Read the model definition and answer for the solid it produces. Units are mm, in the model's axes. A direction names the side the tool comes from. Give positions to 0.01 mm unless a question says otherwise; leave off trailing zeros. Loops run counter-clockwise (first coordinate to the right, second up) from the corner with the lowest first, then second, coordinate; pieces in that order, holes last. Notation, with made-up numbers: (-22, 34) - (7, 34) arc R24 cw to (7, 64) - close; hole circle Ø4 at (32.25, 28). An arc over 180 degrees is marked (long way). Put each result on its own line as item: value. Start each with the question number.
1. A cutting plane is placed at A-A, the plane z = 23. Count the separate pieces of the cut face and the enclosed holes in it, plus the area to 3 significant figures.
2. Given pin 1 Ø4.5 at (x, y) = (15, 5.1) entering from +Z; pin 2 Ø2 at (x, y) = (0, 20.1) entering from +Z; pin 3 Ø5 at (x, z) = (19, 12.5) entering from +Y; pin 4 Ø6 at (x, z) = (-22, 11) entering from -Y, each flat-ended and moving along its own axis, determine where each tip first touches the part or whether it passes through.
3. A cutting plane is placed at B-B, the plane x = -15. Determine the outline of the cut face in (y, z), plus the area to 3 significant figures.
4. For faces 4 (the flat face through (-9.1, -15, 12)), 5 (the cylindrical face through (26.4, 5.23, 0.94)), 6 (the flat face through (-9.1, 25, 12)), 7 (the flat face through (18, 10.2, 13)), determine the directions among +Z, -Z, +X, -X, +Y, -Y from which every point of the face is accessible in a straight line to the end or side of a thin tool.
5. A cutting plane is placed at D-D, the plane y = 20.1. Determine the outline of the cut face in (x, z).
6. For a pull along X with two mould halves and no side action, classify faces 1 (the flat face through (28.484, 12, 12)), 2 (the flat face through (0, 3, 2)), 3 (the flat face through (-20, -4, 12)) as released by +X, released by -X, zero draft, split by the parting line, or undercut.
7. A cutting plane is placed at C-C, the plane y = 5.1. Determine the outline of the cut face in (x, z), plus the area to 3 significant figures.
8. Consider L1, parallel to Y at x = -14.5, z = 9; L2, parallel to X at y = 24, z = 13; L3, parallel to X at y = 20.1, z = 1.65. Determine where each line is inside the solid, lowest interval first. Write a range as from..to.
```python
from build123d import *

# Parameters (mm, degrees)
F1_DEPTH       = 2
F2_DEPTH       = 25
F3_R           = 2
F4_T1_DEPTH    = 4
F4_T3_DEPTH    = 4
F4_T5_DEPTH    = 4
F4_T7_DEPTH    = 18.2
F4_T9_DEPTH    = 18.2
F4_T11_DEPTH   = 4
F5_R           = 2
F6_SIZE        = 2
F8_D           = 3.3
F8_CSINK_D     = 6
F8_CSINK_ANGLE = 90


# Not quite as in the source:
# - a fillet or chamfer that OpenCascade refuses, or shapes differently, is made with other operations: its cross-section is extruded or revolved along the edge and cut away or added
# - a feature names something its author has since deleted; it is built from what else it names


with BuildPart() as f1:
    # F0 (on Top) → F1 (new body)
    with BuildSketch(Plane.XY):
        Polygon((28.4836267311, 0), (28.4836267311, 10.2), (5.1, 10.2), (5.1, 33.5836267311), (-5.1, 33.5836267311), (-5.1, 10.2), (-28.4836267311, 10.2), (-28.4836267311, 0), (-5.1, 0), (-5.1, -23.3836267311), (5.1, -23.3836267311), (5.1, 0), align=None)
        Polygon((5.1, 10.2), (28.4836267311, 10.2), (28.4836267311, 14.2), (9.1, 14.2), (9.1, 33.5836267311), (5.1, 33.5836267311), align=None)
        Polygon((28.4836267311, -4), (28.4836267311, 0), (5.1, 0), (5.1, -23.3836267311), (9.1, -23.3836267311), (9.1, -4), align=None)
        Polygon((-5.1, 10.2), (-5.1, 33.5836267311), (-9.1, 33.5836267311), (-9.1, 14.2), (-28.4836267311, 14.2), (-28.4836267311, 10.2), align=None)
        Polygon((-9.1, -23.3836267311), (-5.1, -23.3836267311), (-5.1, 0), (-28.4836267311, 0), (-28.4836267311, -4), (-9.1, -4), align=None)
    extrude(amount=F1_DEPTH)

    # F0 (on Top) → F2 (join)
    with BuildSketch(Plane.XY):
        Polygon((-5.1, 10.2), (-5.1, 33.5836267311), (-9.1, 33.5836267311), (-9.1, 14.2), (-28.4836267311, 14.2), (-28.4836267311, 10.2), align=None)
        Polygon((5.1, 10.2), (28.4836267311, 10.2), (28.4836267311, 14.2), (9.1, 14.2), (9.1, 33.5836267311), (5.1, 33.5836267311), align=None)
        Polygon((-9.1, -23.3836267311), (-5.1, -23.3836267311), (-5.1, 0), (-28.4836267311, 0), (-28.4836267311, -4), (-9.1, -4), align=None)
        Polygon((28.4836267311, -4), (28.4836267311, 0), (5.1, 0), (5.1, -23.3836267311), (9.1, -23.3836267311), (9.1, -4), align=None)
    extrude(amount=F2_DEPTH)

    # F3
    f3_edges = [f1.edges().sort_by_distance(p)[0] for p in [
        (9.1, 14.2, 12.5),
        (9.1, -4, 12.5),
    ]]
    fillet(f3_edges, radius=F3_R)

    # F4: fillet of radius 5 on 12 edges, made by hand

    # F4_s2 → F4_t1 (cut)
    with BuildSketch(Plane.XZ.offset(-14.2)):
        with BuildLine():
            ThreePointArc((23.4836267311, 25), (27.0191606371, 23.5355339059), (28.4836267311, 20))
            Line((28.4836267311, 20), (28.5836267311, 20))
            Line((28.5836267311, 20), (28.5836267311, 25.1))
            Line((28.5836267311, 25.1), (23.4836267311, 25.1))
            Line((23.4836267311, 25.1), (23.4836267311, 25))
        make_face()
        with BuildLine():
            ThreePointArc((-28.4836267311, 20), (-27.0191606371, 23.5355339059), (-23.4836267311, 25))
            Line((-23.4836267311, 25), (-23.4836267311, 25.1))
            Line((-23.4836267311, 25.1), (-28.5836267311, 25.1))
            Line((-28.5836267311, 25.1), (-28.5836267311, 20))
            Line((-28.5836267311, 20), (-28.4836267311, 20))
        make_face()
    extrude(amount=F4_T1_DEPTH, mode=Mode.SUBTRACT)

    # F4_s4 → F4_t3 (cut)
    with BuildSketch(Plane.YZ.offset(-9.1)):
        with BuildLine():
            ThreePointArc((33.5836267311, 20), (32.1191606371, 23.5355339059), (28.5836267311, 25))
            Line((28.5836267311, 25), (28.5836267311, 25.1))
            Line((28.5836267311, 25.1), (33.6836267311, 25.1))
            Line((33.6836267311, 25.1), (33.6836267311, 20))
            Line((33.6836267311, 20), (33.5836267311, 20))
        make_face()
        with BuildLine():
            ThreePointArc((-23.3836267311, 20), (-21.9191606371, 23.5355339059), (-18.3836267311, 25))
            Line((-18.3836267311, 25), (-18.3836267311, 25.1))
            Line((-18.3836267311, 25.1), (-23.4836267311, 25.1))
            Line((-23.4836267311, 25.1), (-23.4836267311, 20))
            Line((-23.4836267311, 20), (-23.3836267311, 20))
        make_face()
    extrude(amount=F4_T3_DEPTH, mode=Mode.SUBTRACT)

    # F4_s6 → F4_t5 (cut)
    with BuildSketch(Plane.YZ.offset(5.1)):
        with BuildLine():
            ThreePointArc((28.5836267311, 25), (32.1191606371, 23.5355339059), (33.5836267311, 20))
            Line((33.5836267311, 20), (33.6836267311, 20))
            Line((33.6836267311, 20), (33.6836267311, 25.1))
            Line((33.6836267311, 25.1), (28.5836267311, 25.1))
            Line((28.5836267311, 25.1), (28.5836267311, 25))
        make_face()
        with BuildLine():
            ThreePointArc((-18.3836267311, 25), (-21.9191606371, 23.5355339059), (-23.3836267311, 20))
            Line((-23.3836267311, 20), (-23.4836267311, 20))
            Line((-23.4836267311, 20), (-23.4836267311, 25.1))
            Line((-23.4836267311, 25.1), (-18.3836267311, 25.1))
            Line((-18.3836267311, 25.1), (-18.3836267311, 25))
        make_face()
    extrude(amount=F4_T5_DEPTH, mode=Mode.SUBTRACT)

    # F4_s8 → F4_t7 (cut)
    with BuildSketch(Plane.XZ.offset(-14.2)):
        with BuildLine():
            ThreePointArc((-23.4836267311, 0), (-27.0191606371, 1.4644660941), (-28.4836267311, 5))
            Line((-28.4836267311, 5), (-28.5836267311, 5))
            Line((-28.5836267311, 5), (-28.5836267311, -0.1))
            Line((-28.5836267311, -0.1), (-23.4836267311, -0.1))
            Line((-23.4836267311, -0.1), (-23.4836267311, 0))
        make_face()
        with BuildLine():
            ThreePointArc((28.4836267311, 5), (27.0191606371, 1.4644660941), (23.4836267311, 0))
            Line((23.4836267311, 0), (23.4836267311, -0.1))
            Line((23.4836267311, -0.1), (28.5836267311, -0.1))
            Line((28.5836267311, -0.1), (28.5836267311, 5))
            Line((28.5836267311, 5), (28.4836267311, 5))
        make_face()
    extrude(amount=F4_T7_DEPTH, mode=Mode.SUBTRACT)

    # F4_s10 → F4_t9 (cut)
    with BuildSketch(Plane.YZ.offset(-9.1)):
        with BuildLine():
            ThreePointArc((28.5836267311, 0), (32.1191606371, 1.4644660941), (33.5836267311, 5))
            Line((33.5836267311, 5), (33.6836267311, 5))
            Line((33.6836267311, 5), (33.6836267311, -0.1))
            Line((33.6836267311, -0.1), (28.5836267311, -0.1))
            Line((28.5836267311, -0.1), (28.5836267311, 0))
        make_face()
        with BuildLine():
            ThreePointArc((-18.3836267311, 0), (-21.9191606371, 1.4644660941), (-23.3836267311, 5))
            Line((-23.3836267311, 5), (-23.4836267311, 5))
            Line((-23.4836267311, 5), (-23.4836267311, -0.1))
            Line((-23.4836267311, -0.1), (-18.3836267311, -0.1))
            Line((-18.3836267311, -0.1), (-18.3836267311, 0))
        make_face()
    extrude(amount=F4_T9_DEPTH, mode=Mode.SUBTRACT)

    # F4_s12 → F4_t11 (cut)
    with BuildSketch(Plane.XZ):
        with BuildLine():
            ThreePointArc((28.4836267311, 20), (27.0191606371, 23.5355339059), (23.4836267311, 25))
            Line((23.4836267311, 25), (23.4836267311, 25.1))
            Line((23.4836267311, 25.1), (28.5836267311, 25.1))
            Line((28.5836267311, 25.1), (28.5836267311, 20))
            Line((28.5836267311, 20), (28.4836267311, 20))
        make_face()
        with BuildLine():
            ThreePointArc((-28.4836267311, 20), (-27.0191606371, 23.5355339059), (-23.4836267311, 25))
            Line((-23.4836267311, 25), (-23.4836267311, 25.1))
            Line((-23.4836267311, 25.1), (-28.5836267311, 25.1))
            Line((-28.5836267311, 25.1), (-28.5836267311, 20))
            Line((-28.5836267311, 20), (-28.4836267311, 20))
        make_face()
    extrude(amount=F4_T11_DEPTH, mode=Mode.SUBTRACT)

    # F5
    f5_edges = [f1.edges().sort_by_distance(p)[0] for p in [
        (-9.1, 14.2, 12.5),
        (-9.1, -4, 12.5),
    ]]
    fillet(f5_edges, radius=F5_R)

    # F6
    f6_edges = [f1.edges().sort_by_distance(p)[0] for p in [
        (5.1, 10.2, 13.5),
        (-5.1, 10.2, 13.5),
        (5.1, 0, 13.5),
        (-5.1, 0, 13.5),
    ]]
    chamfer(f6_edges, length=F6_SIZE)

    # F8 (through all)
    with Locations(Plane(origin=(0, 0, 0), x_dir=(1, 0, 0), z_dir=(0, 0, -1))):
        with Locations((0, 9.587961331), (-15, -5.1), (15, -5.1), (0, -20.1)):
            CounterSinkHole(F8_D / 2, F8_CSINK_D / 2, counter_sink_angle=F8_CSINK_ANGLE)


solid = f1.part
```
Return value:
1. separate pieces: 4
1. enclosed holes: 0
1. area: 648 mm2
2. pin 1: stops at z = 2
2. pin 2: passes through
2. pin 3: stops at y = 14.2
2. pin 4: stops at y = -4
3. outline: (-4, 0) - (2.1, 0) - (3.45, 1.35) - (3.45, 2) - (0, 2) - (0, 25) - (-4, 25) - close; (6.75, 1.35) - (8.1, 0) - (14.2, 0) - (14.2, 25) - (10.2, 25) - (10.2, 2) - (6.75, 2) - close
3. area: 212 mm2
4. face 4: +Z, -Z, -X, -Y
4. face 5: -Z, +X, +Y, -Y
4. face 6: +Z, -Z, -X, +Y
4. face 7: +Z, +X, -X
5. outline: (-9.1, 0) - (-3, 0) - (-1.65, 1.35) - (-1.65, 2) - (-5.1, 2) - (-5.1, 25) - (-9.1, 25) - close; (1.65, 1.35) - (3, 0) - (9.1, 0) - (9.1, 25) - (5.1, 25) - (5.1, 2) - (1.65, 2) - close
6. face 1: released by +X
6. face 2: undercut
6. face 3: zero draft
7. outline: (-27.48, 2) arc R5 ccw to (-23.48, 0) - (-18, 0) - (-16.65, 1.35) - (-16.65, 2) - close; (-13.35, 1.35) - (-12, 0) - (12, 0) - (13.35, 1.35) - (13.35, 2) - (-13.35, 2) - close; (16.65, 1.35) - (18, 0) - (23.48, 0) arc R5 ccw to (27.48, 2) - (16.65, 2) - close
7. area: 88.3 mm2
8. L1: y = -4..0, 10.2..14.2
8. L2: x = -9.1..-5.1, 5.1..9.1
8. L3: x = -9.1..-1.65, 1.65..9.1
